from build123d import *

# Parameters (mm, degrees)
SCHIZZO1_W                     = 88
SCHIZZO1_H                     = 138
ESTRUSIONE_SOTTILE1_DEPTH      = 1000
ESTRUSIONE1_DEPTH              = 1017.120071645
ESTRUSIONE2_DEPTH              = 1017.120071645
SCHIZZO4_R                     = 30
ESTRUSIONE3_DEPTH              = 1017.120071645
SCHIZZO12_R                    = 7
TAGLIO_ESTRUSIONE1_DEPTH       = 1017.120071645
SCHIZZO5_W                     = 100
SCHIZZO5_H                     = 360
ESTRUSIONE4_DEPTH              = 5
SCHIZZO6_R                     = 7
ESTRUSIONE5_DEPTH              = 1017.870198206
SCHIZZO9_R                     = 30
ESTRUSIONE8_DEPTH              = 1017.870198206
ESTRUSIONE_SOTTILE2_DEPTH      = 260
ESTRUSIONE_SOTTILE2_DEPTH_BACK = 360
SCHIZZO10_R                    = 30
SCHIZZO10_R_2                  = 26
ESTRUSIONE_SOTTILE3_START      = -5
SCHIZZO11_W                    = 94
SCHIZZO11_H                    = 54
ESTRUSIONE_SOTTILE3_DEPTH      = 90


with BuildPart() as part:
    # Schizzo1 → Estrusione-Sottile1 (new body)
    with BuildSketch(Plane.XY):
        with BuildLine():
            Line((5, 0), (95, 0))
            ThreePointArc((95, 0), (98.535533906, 1.464466094), (100, 5))
            Line((100, 5), (100, 145))
            ThreePointArc((100, 145), (98.535533906, 148.535533906), (95, 150))
            Line((95, 150), (5, 150))
            ThreePointArc((5, 150), (1.464466094, 148.535533906), (0, 145))
            Line((0, 145), (0, 5))
            ThreePointArc((0, 5), (1.464466094, 1.464466094), (5, 0))
        make_face()
        with Locations((50, 75)):
            Rectangle(SCHIZZO1_W, SCHIZZO1_H, mode=Mode.SUBTRACT)
    extrude(amount=ESTRUSIONE_SOTTILE1_DEPTH)

    # Schizzo2 → Estrusione1 (cut, through all)
    with BuildSketch(Plane(origin=(100, 0, 0), x_dir=(0, 0, -1), z_dir=(1, 0, 0))):
        Polygon((-920, 0), (-1000, 150), (-1000, 0), align=None)
    extrude(amount=-ESTRUSIONE1_DEPTH, mode=Mode.SUBTRACT)

    # Schizzo3 → Estrusione2 (cut, through all)
    with BuildSketch(Plane(origin=(100, 0, 0), x_dir=(0, 0, -1), z_dir=(1, 0, 0))):
        Polygon((-180, 150), (-260, 0), (0, 0), (0, 150), align=None)
    extrude(amount=-ESTRUSIONE2_DEPTH, mode=Mode.SUBTRACT)

    # Schizzo4 → Estrusione3 (cut, through all)
    with BuildSketch(Plane.XZ):
        with Locations(Location((50, 850, 0), (0, 0, 270))):
            Circle(SCHIZZO4_R)
    extrude(amount=-ESTRUSIONE3_DEPTH, mode=Mode.SUBTRACT)

    # Schizzo12 → Taglio-Estrusione1 (cut, through all)
    with BuildSketch(Plane(origin=(0, 150, 0), x_dir=(1, 0, 0), z_dir=(0, 1, 0))):
        with Locations(Location((50, -693.5, 0), (0, 0, 270))):
            Circle(SCHIZZO12_R)
        with Locations(Location((50, -533.5, 0), (0, 0, 270))):
            Circle(SCHIZZO12_R)
    extrude(amount=-TAGLIO_ESTRUSIONE1_DEPTH, mode=Mode.SUBTRACT)

    # Schizzo5 → Estrusione4 (add)
    with BuildSketch(Plane(origin=(0, 150, 0), x_dir=(1, 0, 0), z_dir=(0, 1, 0))):
        with Locations((50, -600)):
            Rectangle(SCHIZZO5_W, SCHIZZO5_H)
    extrude(amount=ESTRUSIONE4_DEPTH)

    # Schizzo6 → Estrusione5 (cut, through all)
    with BuildSketch(Plane(origin=(0, 155, 0), x_dir=(1, 0, 0), z_dir=(0, 1, 0))):
        with Locations(Location((50, -533.5, 0), (0, 0, 270))):
            Circle(SCHIZZO6_R)
        with Locations(Location((50, -693.5, 0), (0, 0, 270))):
            Circle(SCHIZZO6_R)
    extrude(amount=-ESTRUSIONE5_DEPTH, mode=Mode.SUBTRACT)

    # Schizzo9 → Estrusione8 (cut, through all)
    with BuildSketch(Plane(origin=(100, 0, 0), x_dir=(0, 0, -1), z_dir=(1, 0, 0))):
        with Locations((-933.333333333, 110)):
            Circle(SCHIZZO9_R)
    extrude(amount=-ESTRUSIONE8_DEPTH, mode=Mode.SUBTRACT)

    # Schizzo10 → Estrusione-Sottile2 (add, two sides: drawn at the far end of the back side and taken through both)
    with BuildSketch(Plane(origin=(100, 0, 0), x_dir=(0, 0, -1), z_dir=(1, 0, 0)).offset(-ESTRUSIONE_SOTTILE2_DEPTH_BACK)):
        with Locations((-933.333333333, 110)):
            Circle(SCHIZZO10_R)
        with Locations((-933.333333333, 110)):
            Circle(SCHIZZO10_R_2, mode=Mode.SUBTRACT)
    extrude(amount=ESTRUSIONE_SOTTILE2_DEPTH + ESTRUSIONE_SOTTILE2_DEPTH_BACK)

    # Schizzo11 → Estrusione-Sottile3 (add)
    with BuildSketch(Plane(origin=(100, 0, 0), x_dir=(0, 0, -1), z_dir=(1, 0, 0)).offset(ESTRUSIONE_SOTTILE3_START)):
        with BuildLine():
            Line((-297, 210), (-203, 210))
            ThreePointArc((-203, 210), (-200.878679656, 209.121320344), (-200, 207))
            Line((-200, 207), (-200, 153))
            ThreePointArc((-200, 153), (-200.878679656, 150.878679656), (-203, 150))
            Line((-203, 150), (-297, 150))
            ThreePointArc((-297, 150), (-299.121320344, 150.878679656), (-300, 153))
            Line((-300, 153), (-300, 207))
            ThreePointArc((-300, 207), (-299.121320344, 209.121320344), (-297, 210))
        make_face()
        with Locations((-250, 180)):
            Rectangle(SCHIZZO11_W, SCHIZZO11_H, mode=Mode.SUBTRACT)
    extrude(amount=-ESTRUSIONE_SOTTILE3_DEPTH)


solid = part.part
Geometry: final body of the model. Coordinates: model frame, mm. A direction names the side the tool comes from. Round coordinates to 2 decimals unless told otherwise and drop trailing zeros. Order: outer loops, then holes, each group sorted by start corner. A loop starts at its lowest first (then second) coordinate and runs counter-clockwise, first axis right, second up.
Q1. Section D-D, the plane x = -204. Output: boundary loops of the cut face in (y, z), and give its area (3 significant figures).
Result sheet:
outline: circle Ø60 at (110, 933.33); hole circle Ø52 at (110, 933.33)
area: 704 mm2
Q2. Access query for faces 4 (the face through (95, 151, 246)), 5 (the face through (5, 151, 246)), 6 (the face through (49.384, 111.319, 963.304)). Directions: +Z, -Z, +X, -X, +Y, -Y. A direction counts if a zero-diameter tool reaches every point of the face in a straight line with its end or side. Return the directions, or none.
Result sheet:
face 4: -Z, +X, +Y
face 5: -Z, -X, +Y
face 6: none
Q3. Section B-B, the plane y = 42. Output: boundary loops of the cut face in (x, z), and give its area (3 significant figures).
Result sheet:
outline: (0, 237.6) - (6, 237.6) - (6, 942.4) - (0, 942.4) - close; (94, 237.6) - (100, 237.6) - (100, 942.4) - (94, 942.4) - close
area: 8,460 mm2
Q4. Material intervals for probe 1 along Y at (x, z) = (23.5, 875); probe 2 along X at (y, z) = (76, 597.5); probe 3 along Y at (x, z) = (28, 677), sorted ascending.
Result sheet:
probe 1: y = 0 to 6, 144 to 150
probe 2: x = 0 to 6, 94 to 100
probe 3: y = 0 to 6, 144 to 155
Q5. Mould query, pull axis Y, two halves, no side actions, for faces 1 (the face through (6, 74, 584)), 2 (the face through (49, 155, 597)), 3 (the face through (0, 76, 584)). Classes: released by +Y, released by -Y, zero draft, split by the parting line, or undercut.
Result sheet:
face 1: undercut
face 2: released by +Y
face 3: zero draft
Q6. Pin query (flat end, axial travel): pin 1 (1 mm diameter, centred on x = 64.5, y = 111.5, fed in from +Z); pin 2 (16 mm diameter, centred on x = 32.5, y = 189.5, fed in from +Z); pin 3 (1.5 mm diameter, centred on x = 32.5, y = 153.5, fed in from +Z); pin 4 (8.5 mm diameter, centred on x = 50, z = 693.5, fed in from +Y). Return the tip coordinate at first contact, or that it passes through.
Result sheet:
pin 1: stops at z = 963.32
pin 2: stops at z = 300
pin 3: stops at z = 780
pin 4: passes through
Q7. Section C-C, the plane z = 491.5. Output: boundary loops of the cut face in (x, y), and give its area (3 significant figures).
Result sheet:
outline: (0, 5) arc R5 ccw to (5, 0) - (95, 0) arc R5 ccw to (100, 5) - (100, 145) arc R5 ccw to (95, 150) - (100, 150) - (100, 155) - (0, 155) - (0, 150) - (5, 150) arc R5 ccw to (0, 145) - close; hole (6, 6) - (94, 6) - (94, 144) - (6, 144) - close
area: 3,330 mm2
Q8. Section A-A, the plane z = 850. Output: boundary loops of the cut face in (x, y), and give its area (3 significant figures).
Result sheet:
outline: (0, 5) arc R5 ccw to (5, 0) - (20, 0) - (20, 6) - (6, 6) - (6, 144) - (20, 144) - (20, 150) - (5, 150) arc R5 ccw to (0, 145) - close; (80, 0) - (95, 0) arc R5 ccw to (100, 5) - (100, 145) arc R5 ccw to (95, 150) - (80, 150) - (80, 144) - (94, 144) - (94, 6) - (80, 6) - close
area: 2,110 mm2
